Model file for the job. Use its own axes, mm. Coordinates: 2 decimals unless noted, no trailing zeros. Loops run counter-clockwise (first coordinate to the right, second up) from the corner with the lowest first, then second, coordinate; pieces in that order, holes last.
from build123d import *

# Parameters (mm, degrees)
CROQUIS1_R              = 4.4
SALIENTE_EXTRUIR1_DEPTH = 180
CROQUIS4_R              = 4.4
SALIENTE_EXTRUIR2_DEPTH = 180
CROQUIS5_R              = 4
SALIENTE_EXTRUIR3_DEPTH = 180
CROQUIS6_R              = 4
SALIENTE_EXTRUIR4_DEPTH = 80
CROQUIS7_R              = 4
SALIENTE_EXTRUIR5_DEPTH = 180


with BuildPart() as part:
    # Croquis1 → Saliente-Extruir1 (new body)
    with BuildSketch(Plane(origin=(0, 0, 0), x_dir=(1, 0, 0), z_dir=(0, 1, 0))):
        Circle(CROQUIS1_R)
    extrude(amount=SALIENTE_EXTRUIR1_DEPTH)

    # Croquis4 → Saliente-Extruir2 (add)
    with BuildSketch(Plane(origin=(0, 0, 0), x_dir=(-1, 0, 0), z_dir=(0, -1, 0))):
        Circle(CROQUIS4_R)
    extrude(amount=SALIENTE_EXTRUIR2_DEPTH)

    # Croquis5 → Saliente-Extruir3 (add)
    with BuildSketch(Plane(origin=(0, 0, 0), x_dir=(0, 0, -1), z_dir=(1, 0, 0))):
        Circle(CROQUIS5_R)
    extrude(amount=SALIENTE_EXTRUIR3_DEPTH)

    # Croquis6 → Saliente-Extruir4 (add)
    with BuildSketch(Plane(origin=(0, 0, 0), x_dir=(0, 0, -1), z_dir=(1, 0, 0))):
        Circle(CROQUIS6_R)
    extrude(amount=-SALIENTE_EXTRUIR4_DEPTH)

    # Croquis7 → Saliente-Extruir5 (add)
    with BuildSketch(Plane.XY):
        Circle(CROQUIS7_R)
    extrude(amount=SALIENTE_EXTRUIR5_DEPTH)


solid = part.part
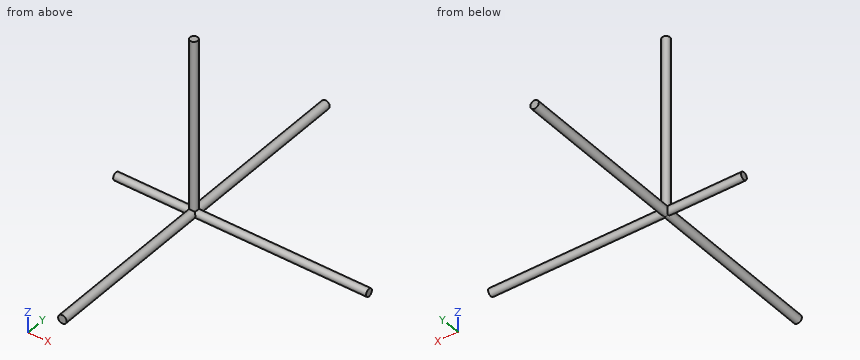
Q1. Slice it at A-A (z = 84). List the corners of the cut face in (x, y).
Answers:
outline: circle Ø8 at (0, 0)
Q2. Drill centre line: line 1 (Z direction, x = -1, y = -161). Where is it in solid material? Low to high.
Answers:
line 1: z = -4.28 to 4.28
Q3. Flat gauge pin, fed straight in: P1, Ø3, axis at y = 7, z = 81, coming from the -X side. Where does the tip first touch, or does it go through?
Answers:
P1: passes through
